Work out the finished part from the listing and answer in its coordinate system (mm). A direction names the side the tool comes from. Coordinates: 2 decimals unless noted, no trailing zeros. Order: outer loops, then holes, each group sorted by start corner. A loop starts at its lowest first (then second) coordinate and runs counter-clockwise, first axis right, second up. Notation, with made-up numbers: M -19.75,-39 L 23.25,-39 A3 cw 23.25,-34 Z; hole C -5,78 d9. An arc over 180 degrees is marked long. Answer in a Markdown table with one row per item. Add a question column.
Item 1: A flat-ended cylindrical pin translates along its axis: pin 1 Ø5 at (x, z) = (0, 0) entering from -Y. Find the tip coordinate at first contact, or state that the pin passes through.
Item 2: The part is cut by section C-C (z = 0). Write down the section's boundary in (x, y).
Item 3: The mould has two halves that part along Z. Classify faces 3 (the face through (-0.77, 1.01, 16.84)), 4 (the face through (7.5, 1, 0)), 5 (the face through (0.088, 1.014, -16.994)), 6 (the face through (0, 1, -20)): released by +Z, released by -Z, zero draft, split by the parting line, or undercut.
Item 4: The part is cut by section B-B (y = 1.45). Write down the section's boundary in (x, z).
Item 5: Consider line 1 (Z direction, x = -0.25, y = 0.2); line 2 (Z direction, x = 1.75, y = 0.5); line 3 (X direction, y = 0.35, z = 15.5). Determine where each line is inside the solid, lowest interval first. Write a range as from..to.
Item 6: The part is cut by section A-A (x = 0). Write down the section's boundary in (y, z), then the cut area to 3 significant figures.
Item 7: Which of the six approach directions +Z, -Z, +X, -X, +Y, -Y give full straight-line access (tool end or side, diameter ignored) to faces 1 (the face through (-7.5, 1, 0)), 2 (the face through (0, 0.5, 0))?
from build123d import *

# Parameters (mm, degrees)
SKETCH2_W           = 15
SKETCH2_H           = 40
BOSS_EXTRUDE1_DEPTH = 2
SKETCH3_R           = 1.5
CUT_EXTRUDE1_DEPTH  = 0.5
SKETCH4_R           = 2
CUT_EXTRUDE2_DEPTH  = 10


with BuildPart() as part:
    # Sketch2 → Boss-Extrude1 (new body)
    with BuildSketch(Plane(origin=(0, 0, 0), x_dir=(1, 0, 0), z_dir=(0, 1, 0))):
        Rectangle(SKETCH2_W, SKETCH2_H)
    extrude(amount=BOSS_EXTRUDE1_DEPTH)

    # Sketch3 → Cut-Extrude1 (cut)
    with BuildSketch(Plane(origin=(0, 0, 0), x_dir=(-1, 0, 0), z_dir=(0, -1, 0))):
        with Locations(Location((0, 0, 0), (0, 0, 90))):
            Circle(SKETCH3_R)
    extrude(amount=-CUT_EXTRUDE1_DEPTH, mode=Mode.SUBTRACT)

    # Sketch4 → Cut-Extrude2 (cut)
    with BuildSketch(Plane(origin=(0, 2, 0), x_dir=(1, 0, 0), z_dir=(0, 1, 0))):
        with Locations(Location((0, 14.995463788, 0), (0, 0, 270))):
            Circle(SKETCH4_R)
        with Locations(Location((0, -14.995463788, 0), (0, 0, 270))):
            Circle(SKETCH4_R)
    extrude(amount=-CUT_EXTRUDE2_DEPTH, mode=Mode.SUBTRACT)


solid = part.part
Reply:
| question | item | result |
|---|---|---|
| 1 | pin 1 | stops at y = 0 |
| 2 | outline | M -7.5,0 L -1.5,0 L -1.5,0.5 L 1.5,0.5 L 1.5,0 L 7.5,0 L 7.5,2 L -7.5,2 Z |
| 3 | face 3 | undercut |
| 3 | face 4 | zero draft |
| 3 | face 5 | undercut |
| 3 | face 6 | released by -Z |
| 4 | outline | M -7.5,-20 L 7.5,-20 L 7.5,20 L -7.5,20 Z; hole C 0,-15 d4; hole C 0,15 d4 |
| 5 | line 1 | z = -20..-16.98, -13.01..-1.48, 1.48..13.01, 16.98..20 |
| 5 | line 2 | z = -20..-15.96, -14.03..14.03, 15.96..20 |
| 5 | line 3 | x = -7.5..-1.94, 1.94..7.5 |
| 6 | outline | M 0,-20 L 2,-20 L 2,-17 L 0,-17 Z; M 0,-13 L 2,-13 L 2,13 L 0,13 L 0,1.5 L 0.5,1.5 L 0.5,-1.5 L 0,-1.5 Z; M 0,17 L 2,17 L 2,20 L 0,20 Z |
| 6 | area | 62.5 mm2 |
| 7 | face 1 | +Z, -Z, -X, +Y, -Y |
| 7 | face 2 | -Y |
